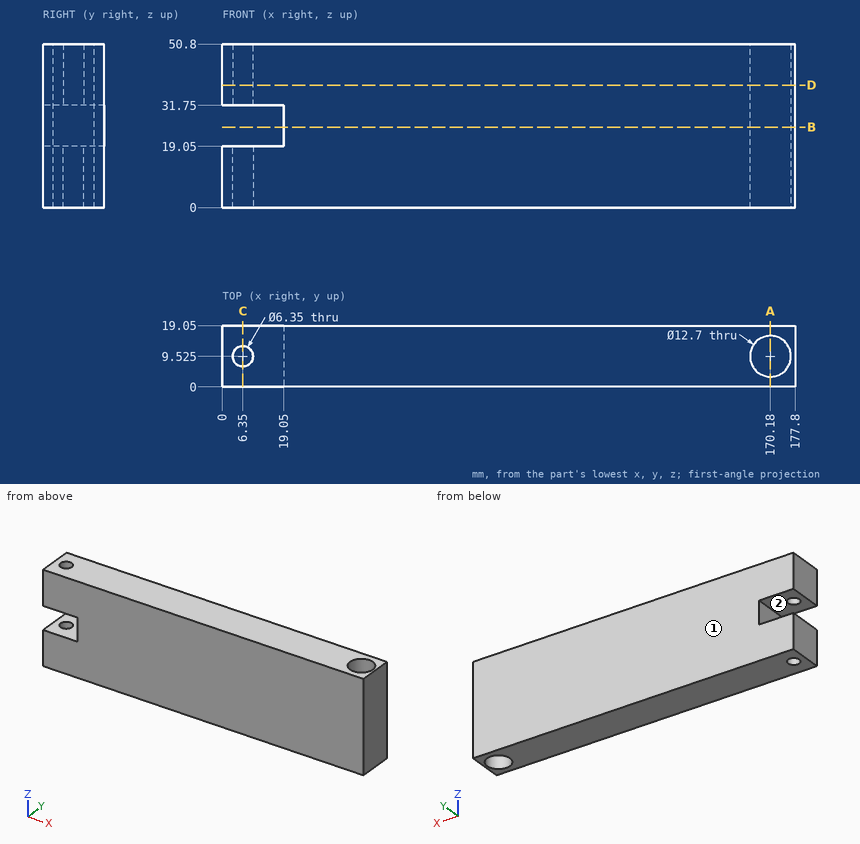
Input: dimensioned drawing with shaded views. Units: mm. Origin: part minimum x, y, z. A direction names the side the tool comes from. Give positions to 0.01 mm unless a question says otherwise; leave off trailing zeros. Order: outer loops, then holes, each group sorted by start corner. A loop starts at its lowest first (then second) coordinate and runs counter-clockwise, first axis right, second up. Notation, with made-up numbers: (-3, 87) -> (45, 87) arc R26 ccw to (45, 116) -> close; hole circle Ø10 at (-19.75, -9.5). An arc over 180 degrees is marked (long way). Use a Markdown table: item, result.
1) Section query D-D, the plane z = 38. Return the cut outline in (x, y) (3 decimals), then the cut area to 3 significant figures.
Answer list:
| item | result |
|---|---|
| outline | (0, 0) -> (177.8, 0) -> (177.8, 19.05) -> (0, 19.05) -> close; hole circle Ø6.35 at (6.35, 9.525); hole circle Ø12.7 at (170.18, 9.525) |
| area | 3,230 mm² |
2) Section query C-C, the plane x = 6.35. Return the cut outline in (y, z), then the cut area to 3 significant figures.
Answer list:
| item | result |
|---|---|
| outline | (0, 0) -> (6.35, 0) -> (6.35, 19.05) -> (0, 19.05) -> close; (0, 31.75) -> (6.35, 31.75) -> (6.35, 50.8) -> (0, 50.8) -> close; (12.7, 0) -> (19.05, 0) -> (19.05, 19.05) -> (12.7, 19.05) -> close; (12.7, 31.75) -> (19.05, 31.75) -> (19.05, 50.8) -> (12.7, 50.8) -> close |
| area | 484 mm² |
3) Reachability of the marked faces 1 and 2 from +Z, -Z, +X, -X, +Y, -Y: full face, straight path, thin tool, end or side. Return the list, or none.
Answer list:
| item | result |
|---|---|
| face 1 | +Z, -Z, +X, -X, +Y |
| face 2 | -X, +Y, -Y |
4) Contact query for flat-ended pins moving along their axis: P1, Ø6.5, axis at y = 7.5, z = 27, coming from the -X side; P2, Ø5, axis at x = 6.35, y = 9.525, coming from the +Z side. Output: stop coordinate, or through.
Answer list:
| item | result |
|---|---|
| P1 | x = 19.05 |
| P2 | through |
5) Ray query, line 1 along Y through (x, z) = (6, 43); line 2 along X through (y, z) = (9, 19); line 3 along X through (y, z) = (11.25, 8). Return the intervals inside material, ascending. Write a range as [from, to].
Answer list:
| item | result |
|---|---|
| line 1 | [0, 6.37], [12.68, 19.05] |
| line 2 | [0, 3.22], [9.48, 163.85], [176.51, 177.8] |
| line 3 | [0, 3.68], [9.02, 164.07], [176.29, 177.8] |
6) Section query B-B, the plane z = 25. Return the cut outline in (x, y) (3 decimals), then the cut area to 3 significant figures.
Answer list:
| item | result |
|---|---|
| outline | (19.05, 0) -> (177.8, 0) -> (177.8, 19.05) -> (19.05, 19.05) -> close; hole circle Ø12.7 at (170.18, 9.525) |
| area | 2,900 mm² |
7) Section query A-A, the plane x = 170.18. Return the cut outline in (y, z) (3 decimals), then the cut area to 3 significant figures.
Answer list:
| item | result |
|---|---|
| outline | (0, 0) -> (3.175, 0) -> (3.175, 50.8) -> (0, 50.8) -> close; (15.875, 0) -> (19.05, 0) -> (19.05, 50.8) -> (15.875, 50.8) -> close |
| area | 323 mm² |
